Could you check a few things on this drawing? It's one solid part, dimensions in mm from its lowest x, y, z. Give positions to 0.01 mm unless a question says otherwise; leave off trailing zeros. Loops run counter-clockwise (first coordinate to the right, second up) from the corner with the lowest first, then second, coordinate; pieces in that order, holes last. Notation, with made-up numbers: M -10.75,-10.5 L 18.25,-10.5 A12 cw 18.25,-5.5 Z; hole C 33,-17.75 d11. An arc over 180 degrees is marked long. Answer as CSV lines item,"result". Start each with the question number.
Item 1: Will this pin go through, and if not, where does the flat tip stop? P1, Ø3.5, axis at x = 15, z = 44, coming from the +Y side.
Item 2: I want a section at C-C on z = 20. List the corners of the cut face in (x, y) for me, plus the area to 3 significant figures.
Item 3: If I drill on line 1 along Z through (x, y) = (133, 0.75); line 2 along X through (y, z) = (0.85, 19); line 3 along X through (y, z) = (1.65, 46), over which ranges is the centre line in solid material (lowest first)? Write a range as from..to.
Item 4: I want a section at D-D on z = 55.5. List the corners of the cut face in (x, y) for me, plus the area to 3 significant figures.
Item 5: I want a section at B-B on x = 15. List the corners of the cut face in (y, z) for me, plus the area to 3 significant figures.
Item 6: I want a section at A-A on y = 2.2. List the corners of the cut face in (x, z) for me, plus the area to 3 significant figures.
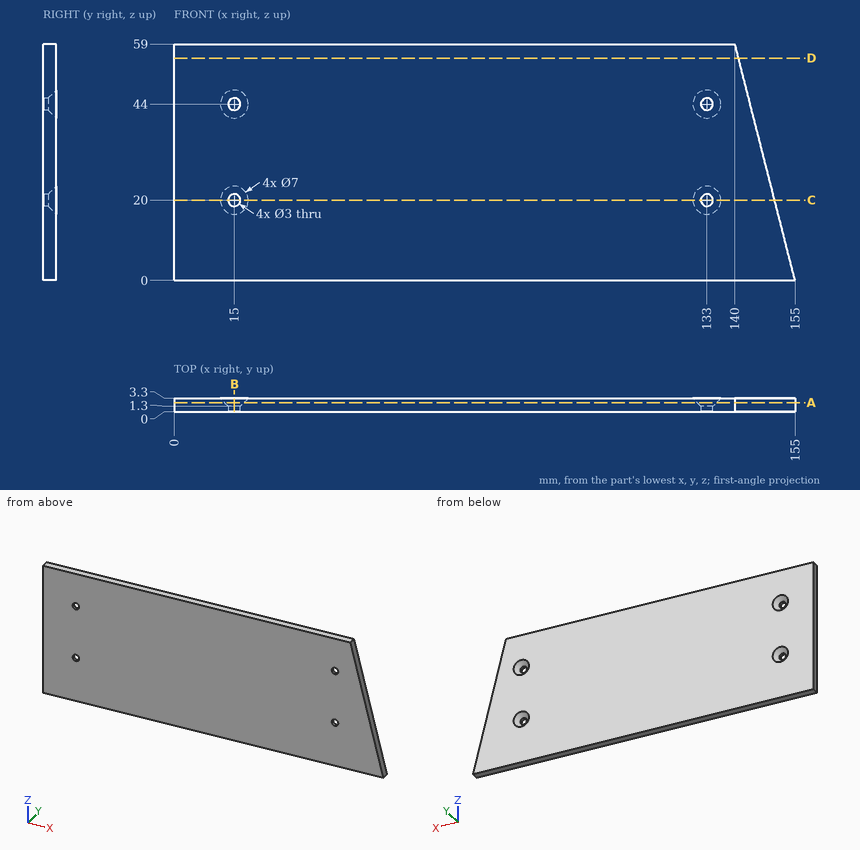
Result:
1,P1,"y = 1.55"
2,outline,"M 0,0 L 13.5,0 L 13.5,1.3 L 11.5,3.3 L 0,3.3 Z; M 16.5,0 L 131.5,0 L 131.5,1.3 L 129.5,3.3 L 18.5,3.3 L 16.5,1.3 Z; M 134.5,0 L 149.92,0 L 149.92,3.3 L 136.5,3.3 L 134.5,1.3 Z"
2,area,"467 mm^2"
3,line 1,"0..18.5, 21.5..42.5, 45.5..59"
3,line 2,"0..13.88, 16.12..131.88, 134.12..150.17"
3,line 3,"0..143.31"
4,outline,"M 0,0 L 140.89,0 L 140.89,3.3 L 0,3.3 Z"
4,area,"465 mm^2"
5,outline,"M 0,0 L 3.3,0 L 3.3,16.5 L 1.3,18.5 L 0,18.5 Z; M 0,21.5 L 1.3,21.5 L 3.3,23.5 L 3.3,40.5 L 1.3,42.5 L 0,42.5 Z; M 0,45.5 L 1.3,45.5 L 3.3,47.5 L 3.3,59 L 0,59 Z"
5,area,"167 mm^2"
6,outline,"M 0,0 L 155,0 L 140,59 L 0,59 Z; hole C 15,20 d4.8; hole C 15,44 d4.8; hole C 133,20 d4.8; hole C 133,44 d4.8"
6,area,"8,630 mm^2"
